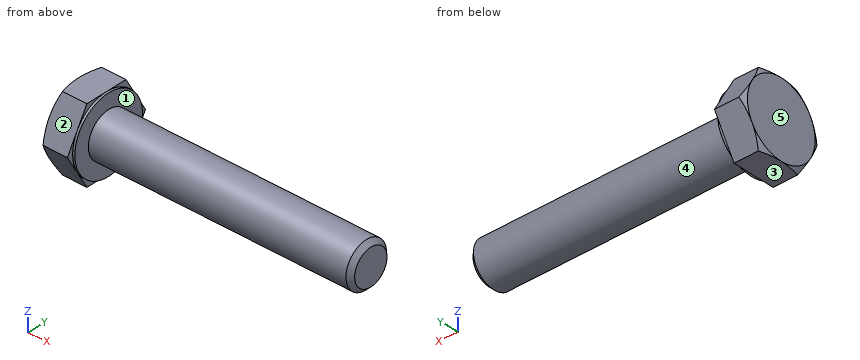
Autodesk Inventor part; units mm, degrees
ref_plane "Work Plane1" through (1.525, 0, 0) normal (0, 0, 1) x (1, 0, 0)
ref_plane "YZ Plane" through (0, 0, 0) normal (1, 0, 0) x (0, 1, 0)
ref_plane "XZ Plane" through (0, 0, 0) normal (0, 1, 0) x (-1, 0, 0)
sketch "Sketch1" plane through (0, 0, 0) normal (0, 0, 1) x (1, 0, 0)
  line L0 (0, 5) -> (0, 3)
  line L1 (17, 3) -> (35, 3)
  line L2 (35, 3) -> (35, 0)
  line L3 (35, 0) -> (-0.3001, 0)
  line L4 (-7.3601, 0) -> (42.06, 0)
  line L5 (-0.3001, 0) -> (-0.3001, 5)
  line L6 (-0.3001, 5) -> (0, 5)
  line L7 (17, 3) -> (16.3865, 3)
  line L8 (16.3865, 3) -> (0, 3)
  line L9 (0, -1) -> (0, 6)
  dimension "d0" = 35
  dimension "d1" = 18
  dimension "d2" = 6
  dimension "d9" = 0.3001
  dimension "d10" = 10
  dimension "d13" = 0.6136
  dimension "d14" = 6
revolve "Body" add sketch "Sketch1" angle 360 about axis through (35, 0, 0) along (-1, 0, 0)
sketch "Sketch2" plane through (-0.3001, 0, 0) normal (-1, 0, 0) x (0, 0, 1)
  line L0 (0, 5.7735) -> (5, 2.8868)
  line L1 (5, 2.8868) -> (5, -2.8868)
  line L2 (5, -2.8868) -> (0, -5.7735)
  line L3 (0, -5.7735) -> (-5, -2.8868)
  line L4 (-5, -2.8868) -> (-5, 2.8868)
  line L5 (-5, 2.8868) -> (0, 5.7735)
  point P0 (0, 0)
  point P1 (0, 0)
  dimension "d11" = 10
extrude "Head" add sketch "Sketch2" along normal blind 3.7
sketch "Sketch4" plane through (0, 0, 0) normal (0, 0, 1) x (1, 0, 0)
  line L0 (-4.0001, 5) -> (-4.0001, 5.7735)
  line L1 (-4.0001, 5.7735) -> (-3.5535, 5.7735)
  line L2 (-3.5535, 5.7735) -> (-4.0001, 5)
  line L3 (-4.7401, 0) -> (0.4399, 0)
  line L4 (-0.3001, 5.7735) -> (-4.0001, 5.7735)
  line L5 (-4.0001, 2.8868) -> (-4.0001, 5.7735)
  dimension "d5" = 30
  dimension "d19" = 10
revolve "Chamfer1" cut sketch "Sketch4" angle 360 about axis through (-10, 0, 0) along (1, 0, 0)
thread "Thread"
chamfer "Chamfer2" distance 0.6135 distance2 0.6136 1 edges at (35, -3, 0) measured on face at (35, 0.7485, -0.6631)
ref_plane "Work Plane1" through (1.525, 0, 0) normal (0, 0, 1) x (1, 0, 0)
equation "\"d11\" = SW"
equation "\"d3\" = KOH - SD"
equation "\"d15\" = GEL"
equation "\"d6\" = -0.5 * SPD + 0.5 * GD"
equation "\"d0\" = NLG"
equation "\"d1\" = GEL"
equation "\"d2\" = GD"
equation "\"d10\" = SD2"
equation "\"d14\" = BDM"
equation "\"d5\" = ANG1"
equation "\"d19\" = SW0"
equation "\"NLG\" = 35"
equation "\"GD\" = NND"
equation "\"BDM\" = NND"
equation "\"KOH\" = 4"
equation "\"GEL\" = 18"
equation "\"SW\" = 10"
equation "\"SW0\" = SW"
equation "\"SPD\" = NND - 1.2269 * PTC"
equation "\"SD2\" = SW"
equation "\"SD\" = WFT"
equation "\"ANG1\" = 30deg"
equation "\"GAL\" = 0.61345 * PTC"
equation "\"GUL\" = 0.61345 * PTC"
equation "\"RR\" = 0.25"
equation "\"WFT\" = 0.3"
equation "\"GD1\" = THREADDIA - 1.2269 * PTC"
equation "\"THREADDIA\" = 6"
equation "\"TOA\" = 30deg"
equation "\"PTC\" = 1"
equation "\"NND\" = 6"
equation "\"E0\" = 1.155 * SW"
properties part number "CNS 3121 - M6 x 35" material "Steel, Mild"
Geometry check sheet. Reference: the model listing, model coordinates, mm. Face numbers are marked on the shaded views. A direction names the side the tool comes from. Coordinates: 2 decimals unless noted, no trailing zeros. Write each loop counter-clockwise with the first axis right and the second up, starting at its lowest first coordinate (ties: lowest second). Pieces come first, ordered by that corner, then holes. Notation, with made-up numbers: M 50.25,12 L 60.25,12 A18 ccw 60.25,39 Z; hole C -19.75,62.5 d5. An arc over 180 degrees is marked long. One line per item, written item: value. Start each with the question number.
(1) Sectioned sample at A-A, the plane x = 3.5. Enter the section's corners in (y, z).
(2) Depth check by flat-ended pin: pin 1 (1.3 mm diameter, centred on y = 1.5, z = -3.5, fed in from +X); pin 2 (2 mm diameter, centred on x = 18, z = -1.5, fed in from -Y); pin 3 (1 mm diameter, centred on x = 18.5, y = 1.5, fed in from -Z); pin 4 (3 mm diameter, centred on y = -2.5, z = -2, fed in from +X). Enter the tip coordinate at first touch or a pass-through.
(3) Release check for a two-part mould opening along Z. For the marked faces 1, 2 and 3 record: released by +Z, released by -Z, zero draft, split by the parting line, or undercut.
(4) Tool access check on the marked faces 4 and 5. Record the directions out of +Z, -Z, +X, -X, +Y, -Y that give a thin tool (end or side, any length) a straight path to the whole face; none if there is none.
(5) Scan lines: line 1 along X through (y, z) = (-2, -4.25); line 2 along Z through (x, y) = (7.5, -1); line 3 along Z through (x, y) = (22, 0.75). Record each from-to range of solid material in increasing order. Write a range as [from, to].
Filled sheet:
1. outline: C 0,0 d6
2. pin 1: x = 0
2. pin 2: y = -2.96
2. pin 3: z = -2.83
2. pin 4: x = 35
3. face 1: zero draft
3. face 2: released by +Z
3. face 3: released by -Z
4. face 4: +X
4. face 5: +Z, -Z, -X, +Y, -Y
5. line 1: [-4, 0]
5. line 2: [-2.83, 2.83]
5. line 3: [-2.9, 2.9]
